```python
from build123d import *

# Parameters (mm, degrees)
BOSS_EXTRUDE1_DEPTH = 3
SKETCH2_R           = 2
BOSS_EXTRUDE2_DEPTH = 2
SKETCH3_R           = 1.1
CUT_EXTRUDE1_DEPTH  = 3.5
SKETCH4_R           = 3
BOSS_EXTRUDE3_DEPTH = 6.12
SKETCH5_R           = 2.1
CUT_EXTRUDE3_DEPTH  = 9.12
SKETCH7_R           = 1.5
BOSS_EXTRUDE4_DEPTH = 2
SKETCH8_R           = 1.2
BOSS_EXTRUDE5_DEPTH = 1
SKETCH9_R           = 0.625
CUT_EXTRUDE6_DEPTH  = 3.5
FILLET2_R           = 0.2


with BuildPart() as part:
    # Sketch1 → Boss-Extrude1 (new body)
    with BuildSketch(Plane(origin=(0, 0, 0), x_dir=(1, 0, 0), z_dir=(0, 1, 0))):
        with BuildLine():
            Line((-11.96, 3), (11.96, 3))
            ThreePointArc((11.96, 3), (14.96, 0), (11.96, -3))
            Line((11.96, -3), (-11.96, -3))
            ThreePointArc((-11.96, -3), (-14.96, 0), (-11.96, 3))
        make_face()
    extrude(amount=BOSS_EXTRUDE1_DEPTH)

    # Sketch2 → Boss-Extrude2 (add)
    with BuildSketch(Plane.XZ):
        with Locations(Location((-11.96, 0, 0), (0, 0, 90))):
            Circle(SKETCH2_R)
    extrude(amount=BOSS_EXTRUDE2_DEPTH)

    # Sketch3 → Cut-Extrude1 (cut)
    with BuildSketch(Plane.XZ.offset(2)):
        with Locations(Location((-11.96, 0, 0), (0, 0, 270))):
            Circle(SKETCH3_R)
    extrude(amount=-CUT_EXTRUDE1_DEPTH, mode=Mode.SUBTRACT)

    # Sketch4 → Boss-Extrude3 (add)
    with BuildSketch(Plane.XZ):
        with Locations(Location((11.96, 0, 0), (0, 0, 270))):
            Circle(SKETCH4_R)
    extrude(amount=BOSS_EXTRUDE3_DEPTH)

    # Sketch5 → Cut-Extrude3 (cut)
    with BuildSketch(Plane.XZ.offset(6.12)):
        with Locations(Location((11.96, 0, 0), (0, 0, 270))):
            Circle(SKETCH5_R)
    extrude(amount=-CUT_EXTRUDE3_DEPTH, mode=Mode.SUBTRACT)

    # Sketch7 → Boss-Extrude4 (add)
    with BuildSketch(Plane(origin=(0, 3, 0), x_dir=(1, 0, 0), z_dir=(0, 1, 0))):
        with Locations(Location((0, 0, 0), (0, 0, 270))):
            Circle(SKETCH7_R)
    extrude(amount=BOSS_EXTRUDE4_DEPTH)

    # Sketch8 → Boss-Extrude5 (add)
    with BuildSketch(Plane(origin=(0, 5, 0), x_dir=(1, 0, 0), z_dir=(0, 1, 0))):
        with Locations(Location((0, 0, 0), (0, 0, 270))):
            Circle(SKETCH8_R)
    extrude(amount=BOSS_EXTRUDE5_DEPTH)

    # Sketch9 → Cut-Extrude6 (cut)
    with BuildSketch(Plane(origin=(0, 6, 0), x_dir=(1, 0, 0), z_dir=(0, 1, 0))):
        with Locations(Location((0, 0, 0), (0, 0, 270))):
            Circle(SKETCH9_R)
    extrude(amount=-CUT_EXTRUDE6_DEPTH, mode=Mode.SUBTRACT)

    # Fillet2
    fillet2_edges = [part.edges().sort_by_distance(p)[0] for p in [
        (0, 6, -1.2),
    ]]
    fillet(fillet2_edges, radius=FILLET2_R)


solid = part.part
```
Geometry check sheet. Reference: the model listing, model coordinates, mm. A direction names the side the tool comes from. Round coordinates to 2 decimals unless told otherwise and drop trailing zeros. Loops run counter-clockwise (first coordinate to the right, second up) from the corner with the lowest first, then second, coordinate; pieces in that order, holes last. Notation, with made-up numbers: (70, 13) - (98, 13) arc R19 cw to (98, 29) - close; hole circle Ø8 at (-39.5, 13). An arc over 180 degrees is marked (long way). Write each question's results on one line, items separated by ' | '. Start each with the question number.
Q1. Cross-section at D-D on y = 2. Enter the section's corners in (x, z), and give its area (3 significant figures).
Q2. Cross-section at B-B on y = -1.5. Enter the section's corners in (x, z).
Q3. Thickness scan on line 1 (X direction, y = -1.25, z = 0); line 2 (X direction, y = 4.25, z = 0) (3 decimals); line 3 (X direction, y = 0.75, z = 0.9). Record the ranges inside material, lowest first. Write a range as [from, to].
Q4. Access from +Z, -Z, +X, -X, +Y, -Y to the whole of each face (thin tool, end or side, straight path). Record for faces 4 (the cylindrical face through (-14.96, 1.48, 0.07)), 5 (the cylindrical face through (-0.61, 4.27, -0.14)), 6 (the cylindrical face through (-12, -1, -2)), 7 (the flat face through (-11, -2, 1)).
Q5. Cross-section at C-C on x = 0. Enter the section's corners in (y, z) (3 decimals).
Q6. Release check for a two-part mould opening along Z. For faces 1 (the flat face through (0, 2.5, 0)), 2 (the flat face through (14, -6.12, -1)), 3 (the cylindrical face through (1.01, 5.39, 0.65)) record: +Z half, -Z half, draft (parallel to the pull), parting line (faces both ways), or undercut.
Q7. Gauge pin test, flat ends, axial feed: P1, Ø1.5, axis at x = -3, z = 1.5, coming from the +Y side; P2, Ø1.6, axis at x = 0, z = 0, coming from the -Y side; P3, Ø2, axis at x = -12, z = 0, coming from the -Y side. Record the tip position at first contact, or that the pin passes through.
Answers below:
1) outline: (-11.96, -3) - (11.96, -3) arc R3 ccw to (11.96, 3) - (-11.96, 3) arc R3 ccw to start; hole circle Ø4.2 at (11.96, 0) | area: 158 mm²
2) outline: circle Ø4 at (-11.96, 0); circle Ø6 at (11.96, 0); hole circle Ø2.2 at (-11.96, 0); hole circle Ø4.2 at (11.96, 0)
3) line 1: x = [-13.96, -13.06], [-10.86, -9.96], [8.96, 9.86], [14.06, 14.96] | line 2: x = [-1.5, -0.625], [0.625, 1.5] | line 3: x = [-14.82, -12.59], [-11.33, 10.06], [13.86, 14.82]
4) face 4: -X, +Y, -Y | face 5: +Y | face 6: -Y | face 7: +Z, -Z, -X, -Y
5) outline: (0, -3) - (3, -3) - (3, -1.5) - (5, -1.5) - (5, -1.2) - (5.8, -1.2) arc R0.2 ccw to (6, -1) - (6, -0.625) - (2.5, -0.625) - (2.5, 0.625) - (6, 0.625) - (6, 1) arc R0.2 ccw to (5.8, 1.2) - (5, 1.2) - (5, 1.5) - (3, 1.5) - (3, 3) - (0, 3) - close
6) face 1: undercut | face 2: draft | face 3: parting line
7) P1: stops at y = 3 | P2: stops at y = 0 | P3: stops at y = 1.5
